from build123d import *

# Parameters (mm, degrees)
SKETCH_1_R          = 0.5
EXTRUDE_1_DEPTH     = 1
SKETCH_3_R          = 0.5
EXTRUDE_2_DEPTH     = 5.5
SKETCH_4_R          = 4.5
EXTRUDE_3_DEPTH     = 3.3
EXTRUDE_4_DEPTH     = 3.6
SKETCH_6_W          = 3
SKETCH_6_H          = 9.3
SKETCH_6_W_2        = 0.5
CUT_EXTRUDE_1_DEPTH = 3


with BuildPart() as part:
    # 草图1 → 凸台-拉伸1 (new body)
    # profile 1 of 2: a face of its own
    with BuildSketch(Plane.XY):
        with BuildLine():
            Line((5, -3.406244266), (5, 3.406244266))
            ThreePointArc((5, 3.406244266), (0, 6.05), (-5, 3.406244266))
            Line((-5, 3.406244266), (-5, -3.406244266))
            ThreePointArc((-5, -3.406244266), (0, -6.05), (5, -3.406244266))
        make_face()
        Circle(SKETCH_1_R, mode=Mode.SUBTRACT)
    # profile 2 of 2: a face of its own
    with BuildSketch(Plane.XY):
        with BuildLine():
            Line((13.35, 6.05), (0, 6.05))
            ThreePointArc((0, 6.05), (2.827960589, 5.348377222), (5, 3.406244266))
            Line((5, 3.406244266), (5, -3.406244266))
            ThreePointArc((5, -3.406244266), (2.827960589, -5.348377222), (0, -6.05))
            Line((0, -6.05), (13.35, -6.05))
            Line((13.35, -6.05), (13.35, 6.05))
        make_face()
    extrude(amount=EXTRUDE_1_DEPTH)

    # 草图3 → 凸台-拉伸2 (add)
    with BuildSketch(Plane(origin=(0, 0, 0), x_dir=(-1, 0, 0), z_dir=(0, 0, -1))):
        Circle(SKETCH_3_R)
    extrude(amount=-EXTRUDE_2_DEPTH)

    # 草图4 → 凸台-拉伸3 (add)
    with BuildSketch(Plane.XY.offset(2)):
        Circle(SKETCH_4_R)
    extrude(amount=EXTRUDE_3_DEPTH)

    # 草图5 → 凸台-拉伸4 (add)
    with BuildSketch(Plane.XY.offset(1)):
        Polygon((13.35, 0), (13.35, 5.15), (9.35, 5.15), (9.35, -5.15), (13.35, -5.15), align=None)
    extrude(amount=EXTRUDE_4_DEPTH)

    # 草图6 → 切除-拉伸1 (cut)
    with BuildSketch(Plane.XY.offset(1)):
        with Locations((11.35, 0)):
            Rectangle(SKETCH_6_W, SKETCH_6_H)
        with Locations((13.1, 0)):
            Rectangle(SKETCH_6_W_2, SKETCH_6_H)
    extrude(amount=CUT_EXTRUDE_1_DEPTH, mode=Mode.SUBTRACT)


solid = part.part
For this review, take the finished solid that the model builds, in its own axes (mm). A direction names the side the tool comes from. Coordinates: 2 decimals unless noted, no trailing zeros. Order: outer loops, then holes, each group sorted by start corner. A loop starts at its lowest first (then second) coordinate and runs counter-clockwise, first axis right, second up. Notation, with made-up numbers: (69.5, 24.5) - (115.5, 24.5) arc R21 cw to (115.5, 45.5) - close; hole circle Ø10 at (59.5, 73.5). An arc over 180 degrees is marked (long way). Use one line per item in the form item = value.
Q1. For P1, Ø0.9, axis at x = 12, z = 2, coming from the +Y side; P2, Ø3, axis at x = 12.5, y = -0.5, coming from the +Z side; P3, Ø1.8, axis at y = 0, z = 2, coming from the -X side, all flat-tipped, find the tip position at first contact; note any pin that passes through.
Checked values:
P1 = 5.15
P2 = 4.6
P3 = -4.5
Q2. Draft analysis for pull direction Y (two halves, no side actions). For faces 6 (the flat face through (12, -4.65, 2)), 7 (the cylindrical face through (-2.79, 5.37, 0.49)), 8 (the flat face through (0, -1, 5.3)), 9 (the flat face through (12, 4.65, 2)), state which applies: +Y half, -Y half, draft (parallel to the pull), parting line (faces both ways), or undercut.
Checked values:
face_6 = undercut
face_7 = +Y half
face_8 = draft
face_9 = undercut
Q3. For probe 1 along Z at (x, y) = (11.5, 2.75); probe 2 along Z at (x, y) = (2.25, -2.5); probe 3 along Z at (x, y) = (-3.75, -4), list the stretches that pass through material, from the lowest coordinate up. Write a range as from..to.
Checked values:
probe_1 = 0..1, 4..4.6
probe_2 = 0..1, 2..5.3
probe_3 = 0..1
Q4. For faces 1 (the flat face through (11, 0, 4.6)), 2 (the flat face through (12, 0, 1)), 3 (the flat face through (11, -5.15, 3)), 4 (the cylindrical face through (0.108, -0.488, 1.493)), 5 (the flat face through (9.35, 0, 3)), list the 3-axis set-ups (+Z, -Z, +X, -X, +Y, -Y) from which the entire face can be reached by the end or side of a thin tool; tool diameter is ignored.
Checked values:
face_1 = +Z, +X, +Y, -Y
face_2 = +X
face_3 = +Z, +X, -X, -Y
face_4 = none
face_5 = +Z, +Y, -Y
Q5. Consider section A-A (z = 2.2). Give the boundary of the cut face in (x, y).
Checked values:
outline = circle Ø9 at (0, 0); (9.35, -5.15) - (13.35, -5.15) - (13.35, -4.65) - (9.85, -4.65) - (9.85, 4.65) - (13.35, 4.65) - (13.35, 5.15) - (9.35, 5.15) - close
Q6. Consider section C-C (x = 8.75). Give the boundary of the cut face in (y, z), then the cut area to 3 significant figures.
Checked values:
outline = (-6.05, 0) - (6.05, 0) - (6.05, 1) - (-6.05, 1) - close
area = 12.1 mm2
Q7. Consider section B-B (y = 4.25). Give the boundary of the cut face in (x, z).
Checked values:
outline = (-4.31, 0) - (13.35, 0) - (13.35, 1) - (9.85, 1) - (9.85, 4) - (13.35, 4) - (13.35, 4.6) - (9.35, 4.6) - (9.35, 1) - (-4.31, 1) - close; (-1.48, 2) - (1.48, 2) - (1.48, 5.3) - (-1.48, 5.3) - close
Q8. Consider section D-D (y = 0). Give the boundary of the cut face in (x, z), then the cut area to 4 significant figures.
Checked values:
outline = (-5, 0) - (13.35, 0) - (13.35, 1) - (9.85, 1) - (9.85, 4) - (13.35, 4) - (13.35, 4.6) - (9.35, 4.6) - (9.35, 1) - (0.5, 1) - (0.5, 2) - (4.5, 2) - (4.5, 5.3) - (0.5, 5.3) - (0.5, 5.5) - (-0.5, 5.5) - (-0.5, 5.3) - (-4.5, 5.3) - (-4.5, 2) - (-0.5, 2) - (-0.5, 1) - (-5, 1) - close
area = 53.15 mm2
